Autodesk Inventor part; units mm, degrees
ref_plane "YZ Plane" through (0, 0, 0) normal (1, 0, 0) x (0, 1, 0)
ref_plane "XZ Plane" through (0, 0, 0) normal (0, 1, 0) x (-1, 0, 0)
ref_plane "XY Plane" through (0, 0, 0) normal (0, 0, 1) x (1, 0, 0)
sketch "Sketch1" plane through (0, 0, 0) normal (0, 1, 0) x (-1, 0, 0)
  circle A0 centre (0, 0) radius 18.5
  dimension "d0" = 37
extrude "Extrusion1" add sketch "Sketch1" along normal blind 7.35
sketch "Sketch2" plane through (0, 7.35, 0) normal (0, 1, 0) x (1, 0, 0)
  circle A0 centre (0, 0) radius 16.665
  dimension "d3" = 33.33
extrude "Extrusion2" cut sketch "Sketch2" against normal blind 4.18
sketch "Sketch3" plane through (0, 0, 0) normal (0, -1, 0) x (1, 0, 0)
  circle A0 centre (0, 0) radius 17
  dimension "d6" = 34
extrude "Extrusion3" add sketch "Sketch3" along normal blind 33
sketch "Sketch4" plane through (0, -33, 0) normal (0, -1, 0) x (1, 0, 0)
  circle A0 centre (0, 0) radius 14.5
  dimension "d9" = 29
extrude "Extrusion4" add sketch "Sketch4" along normal blind 3.9
sketch "Sketch5" plane through (0, -36.9, 0) normal (0, -1, 0) x (1, 0, 0)
  circle A0 centre (0, 0) radius 12.7
  dimension "d12" = 25.4
extrude "Extrusion5" add sketch "Sketch5" along normal blind 5.65
thread "Thread1"
sketch "Sketch6" plane through (0, 3.17, 0) normal (0, 1, 0) x (1, 0, 0)
  circle A0 centre (0, 0) radius 11
  dimension "d17" = 22
extrude "Extrusion6" cut sketch "Sketch6" against normal blind 1
properties part number "Tamron_M118M06"
Read the model definition and answer for the solid it produces. Units are mm, in the model's axes. A direction names the side the tool comes from. Coordinates: 2 decimals unless noted, no trailing zeros. Loops run counter-clockwise (first coordinate to the right, second up) from the corner with the lowest first, then second, coordinate; pieces in that order, holes last.
(1) The part is cut by section A-A (x = 3). Determine the outline of the cut face in (y, z).
Solution:
outline: (-42.55, -12.34) - (-36.9, -12.34) - (-36.9, -14.19) - (-33, -14.19) - (-33, -16.73) - (0, -16.73) - (0, -18.26) - (7.35, -18.26) - (7.35, -16.39) - (3.17, -16.39) - (3.17, -10.58) - (2.17, -10.58) - (2.17, 10.58) - (3.17, 10.58) - (3.17, 16.39) - (7.35, 16.39) - (7.35, 18.26) - (0, 18.26) - (0, 16.73) - (-33, 16.73) - (-33, 14.19) - (-36.9, 14.19) - (-36.9, 12.34) - (-42.55, 12.34) - close
(2) Consider line 1 along Z through (x, y) = (0, 6) (3 decimals); line 2 along Y through (x, z) = (10.5, 6); line 3 along Z through (x, y) = (0, 2.55). Determine where each line is inside the solid, lowest interval first.
Solution:
line 1: z = -18.5 to -16.665, 16.665 to 18.5
line 2: y = -42.55 to 3.17
line 3: z = -18.5 to -11, 11 to 18.5
(3) The mould has two halves that part along X. Classify faces 4 (the face through (0, 2.17, 0)), 5 (the face through (13, -33, 8)), 6 (the face through (-2.75, -39.69, 12.4)): released by +X, released by -X, zero draft, split by the parting line, or undercut.
Solution:
face 4: undercut
face 5: zero draft
face 6: split by the parting line
(4) The part is cut by section B-B (z = 0). Determine the outline of the cut face in (x, y) (3 decimals).
Solution:
outline: (-18.5, 0) - (-17, 0) - (-17, -33) - (-14.5, -33) - (-14.5, -36.9) - (-12.7, -36.9) - (-12.7, -42.55) - (12.7, -42.55) - (12.7, -36.9) - (14.5, -36.9) - (14.5, -33) - (17, -33) - (17, 0) - (18.5, 0) - (18.5, 7.35) - (16.665, 7.35) - (16.665, 3.17) - (11, 3.17) - (11, 2.17) - (-11, 2.17) - (-11, 3.17) - (-16.665, 3.17) - (-16.665, 7.35) - (-18.5, 7.35) - close
(5) Flat-ended cylindrical pins translate along their axes: pin 1 Ø5 at (x, z) = (-1.5, 11.5) entering from +Y; pin 2 Ø1.5 at (y, z) = (-11, 9) entering from -X; pin 3 Ø10 at (y, z) = (-1.5, 9.5) entering from +X (3 decimals). Find the tip coordinate at first contact, or state that the pin passes through.
Solution:
pin 1: stops at y = 3.17
pin 2: stops at x = -14.86
pin 3: stops at x = 17.885
(6) The part is cut by section C-C (y = -38.5). Determine the outline of the cut face in (x, z).
Solution:
outline: circle Ø25.4 at (0, 0)
(7) The part is cut by section D-D (y = -3). Determine the outline of the cut face in (x, z).
Solution:
outline: circle Ø34 at (0, 0)
(8) A tool of negligible diameter and unlimited length cuts with its end or side. For faces 1 (the face through (0, -36.9, -13)), 2 (the face through (-3.61, 5.29, 16.27)), 3 (the face through (4.01, 3.62, 18.06)), from which of +Z, -Z, +X, -X, +Y, -Y can it reach the whole face along a straight path? Write none if from no direction.
Solution:
face 1: -Y
face 2: +Y
face 3: +Y, -Y
